Can you work these out from the model? Positions are in its coordinate system, mm. A direction names the side the tool comes from. Give positions to 0.01 mm unless a question says otherwise; leave off trailing zeros. Write each loop counter-clockwise with the first axis right and the second up, starting at its lowest first coordinate (ties: lowest second). Pieces come first, ordered by that corner, then holes. Notation, with made-up numbers: (-33, 52) -> (-28, 52) arc R20 ccw to (-28, 78) -> close; hole circle Ø8 at (76.5, -13.75). An arc over 180 degrees is marked (long way). One line per item, written item: value.
Autodesk Inventor part; units mm, degrees
ref_plane "Work Plane1" through (-2, -14.8661, 0) normal (0, 1, 0) x (1, 0, 0)
ref_plane "YZ Plane" through (0, 0, 0) normal (1, 0, 0) x (0, 1, 0)
ref_plane "XZ Plane" through (0, 0, 0) normal (0, 1, 0) x (-1, 0, 0)
sketch "Sketch1" plane through (0, 0, 0) normal (0, 0, 1) x (1, 0, 0)
  arc A0 (-14.4568, -4) -> (14.4568, -4) centre (0, 0) ccw
  circle A1 centre (0, 0) radius 5.5
  line L0 (0, 0) -> (0, -4)
  line L1 (-5.5, 0) -> (-14.4568, -4)
  line L2 (5.5, 0) -> (14.4568, -4)
  line L3 (0, 0) -> (0, 8)
  circle A2 centre (0, 8) radius 2
  line L4 (-5.4025, 1.0312) -> (-3.9291, 8.75)
  line L5 (3.9291, 8.75) -> (5.4025, 1.0313)
  arc A3 (3.9291, 8.75) -> (-3.9291, 8.75) centre (0, 8) ccw
  line L6 (-2, 14.8661) -> (2, 14.8661)
  line L7 (2, 14.8661) -> (2, -14.8661)
  line L8 (2, -14.8661) -> (-2, -14.8661)
  line L9 (-2, -14.8661) -> (-2, 14.8661)
  line L10 (-2, 14.8661) -> (2, -14.8661) construction
  line L11 (2, 14.8661) -> (-2, -14.8661) construction
  dimension "d0" = 30
  dimension "d1" = 11
  dimension "d2" = 4
  dimension "d3" = 8
  dimension "d4" = 4
extrude "Extrusion1" add sketch "Sketch1" along normal blind 6 contours L1 A1 L9 A0 | L8 A0 | L9 A1 L7 L8 | A1 L9 | L7 A1 L2 A0 | L9 A1 L7 | L4 A3 L9 A1 | L7 A1 | L9 A2 L3 A1 | L7 A3 L5 A1 | A1 L3 A2 L7 | L9 A3 L7 A2
sketch "Sketch2" plane through (0, 0, 6) normal (0, 0, 1) x (1, 0, 0)
  arc A0 (5.5, 0) -> (5.4025, 1.0313) centre (0, 0) ccw
  circle A1 centre (0, 0) radius 5.5
  point P0 (5.4025, 1.0313)
extrude "Extrusion2" add sketch "Sketch2" along normal blind 0.5
sketch "Sketch3" plane through (0, 0, 6.5) normal (0, 0, 1) x (1, 0, 0)
  point P0 (0, 0)
hole "Hole2" at (0, 0, 6.5) direction (0, 0, -1) diameter 8 end through all
sketch "Sketch4" plane through (0, 0, 6) normal (0, 0, 1) x (1, 0, 0)
  point P0 (0, 0)
ref_plane "Work Plane1" through (-2, -14.8661, 0) normal (0, 1, 0) x (1, 0, 0)
sketch "Sketch5" plane through (-2, -14.8661, 0) normal (0, 1, 0) x (1, 0, 0)
  line L0 (4, -6) -> (0, -6)
  line L1 (2, -6) -> (2, -3)
  point P0 (2, 0)
  dimension "d26" = 3
hole "Hole3" at (0, -14.8661, 3) direction (0, 1, 0) diameter 4 depth 11 tip angle 118
sketch "Sketch6" plane through (-2, -14.8661, 0) normal (0, 1, 0) x (1, 0, 0)
  arc A0 (4, -3) -> (0, -3) centre (2, -3) ccw
  circle A1 centre (2, -3) radius 2
  point P0 (2, 0)
hole "Hole4" at (0, -14.8661, 3) direction (0, -1, 0) diameter 4 depth 11 tip angle 118
properties part number "KURBEL PART 8"
1) If we section it at C-C (y = -6.5): Write out the boundary of the cut face in (x, z), and give its area (3 significant figures).
Answer list:
outline: (-13.52, 0) -> (13.52, 0) -> (13.52, 6) -> (-13.52, 6) -> close; hole circle Ø4 at (0, 3)
area: 150 mm^2
2) If we section it at B-B (y = 2): Write out the boundary of the cut face in (x, z), and give its area (3 significant figures).
Answer list:
outline: (-5.22, 0) -> (-3.46, 0) -> (-3.46, 6.5) -> (-5.12, 6.5) -> (-5.12, 6) -> (-5.22, 6) -> close; (3.46, 0) -> (5.22, 0) -> (5.22, 6) -> (5.12, 6) -> (5.12, 6.5) -> (3.46, 6.5) -> close
area: 22.7 mm^2
3) If we section it at D-D (y = 7.5): Write out the boundary of the cut face in (x, z).
Answer list:
outline: (-4.17, 0) -> (-1.94, 0) -> (-1.94, 6) -> (-4.17, 6) -> close; (1.94, 0) -> (4.17, 0) -> (4.17, 6) -> (1.94, 6) -> close
4) I need wall thicknesses on L1, parallel to Y at x = 0, z = 1.75; L2, parallel to Y at x = -0.5, z = 5.5; L3, parallel to Z at x = -13, y = -3.5. Which ranges of each line are inside material? Lowest first, please.
Answer list:
L1: y = 4 to 6, 10 to 12
L2: y = -14.99 to -3.97, 3.97 to 6.06, 9.94 to 11.97
L3: z = 0 to 6
5) If we section it at A-A (x = 0): Write out the boundary of the cut face in (y, z).
Answer list:
outline: (-15, 0) -> (-4, 0) -> (-4, 1) -> (-15, 1) -> close; (-15, 5) -> (-4, 5) -> (-4, 6.5) -> (-5.5, 6.5) -> (-5.5, 6) -> (-15, 6) -> close; (4, 0) -> (6, 0) -> (6, 6) -> (5.5, 6) -> (5.5, 6.5) -> (4, 6.5) -> close; (10, 0) -> (12, 0) -> (12, 6) -> (10, 6) -> close
6) For faces 5 (the face through (-0.2, -4.3, 0)), 6 (the face through (1.82, -3.76, 2.97)), 7 (the face through (-5.462, 0.643, 5.161)), which set-ups out of +Z, -Z, +X, -X, +Y, -Y let a thin tool reach every point of the face, with its end or its side?
Answer list:
face 5: -Z, +X, -X, +Y, -Y
face 6: -Y
face 7: +Z
7) We'd pull the mould along X, two halves only. Please class faces 1 (the face through (-0.74, -9.36, 1.14)), 2 (the face through (0, 6, 3)), 3 (the face through (-4.676, 4.837, 2.958)), 4 (the face through (5.475, 0.525, 2.958)): released by +X, released by -X, zero draft, split by the parting line, or undercut.
Answer list:
face 1: undercut
face 2: undercut
face 3: released by -X
face 4: released by +X
8) Will these pins go through, and if not, where does the flat tip stop? pin 1 (2 mm diameter, centred on y = 5.5, z = 2.5, fed in from +X); pin 2 (2 mm diameter, centred on y = 0.5, z = 1.5, fed in from -X).
Answer list:
pin 1: stops at x = 4.74
pin 2: stops at x = -6.62
